Check sheet for the drawn part. Datum: minimum x, y, z corner. Units: mm. A direction names the side the tool comes from. Give positions to 0.01 mm unless a question says otherwise; leave off trailing zeros. Loops run counter-clockwise (first coordinate to the right, second up) from the corner with the lowest first, then second, coordinate; pieces in that order, holes last.
1. Cross-section at B-B, the plane y = 9.5. Record the cut outline in (x, z).
2. Material ranges on L1, parallel to Z at x = 21, y = 1.05; L2, parallel to X at y = 15.3, z = 13 (1 decimal); L3, parallel to Y at x = 3.5, z = 19, recorded low to high.
3. Go/stop test with flat-tipped pins: pin 1 Ø6 at (x, z) = (34.86, 13) entering from -Y; pin 2 Ø3 at (x, y) = (23.5, 7) entering from +Z; pin 3 Ø6 at (x, y) = (9.5, 7.5) entering from +Z. Record where each tip stops, or that it passes through.
4. Tool access check on the marked faces 1 and 2. Record the directions out of +Z, -Z, +X, -X, +Y, -Y that give a thin tool (end or side, any length) a straight path to the whole face; none if there is none.
5. Cross-section at A-A, the plane z = 21. Record the cut outline in (x, y).
6. Release check for a two-part mould opening along X. For the marked faces 3 and 4 record: +X half, -X half, draft (parallel to the pull), parting line (faces both ways), or undercut.
7. Cross-section at C-C, the plane z = 36. State how many separate pieces and enclosed holes the cut face has, plus the area to 3 significant figures.
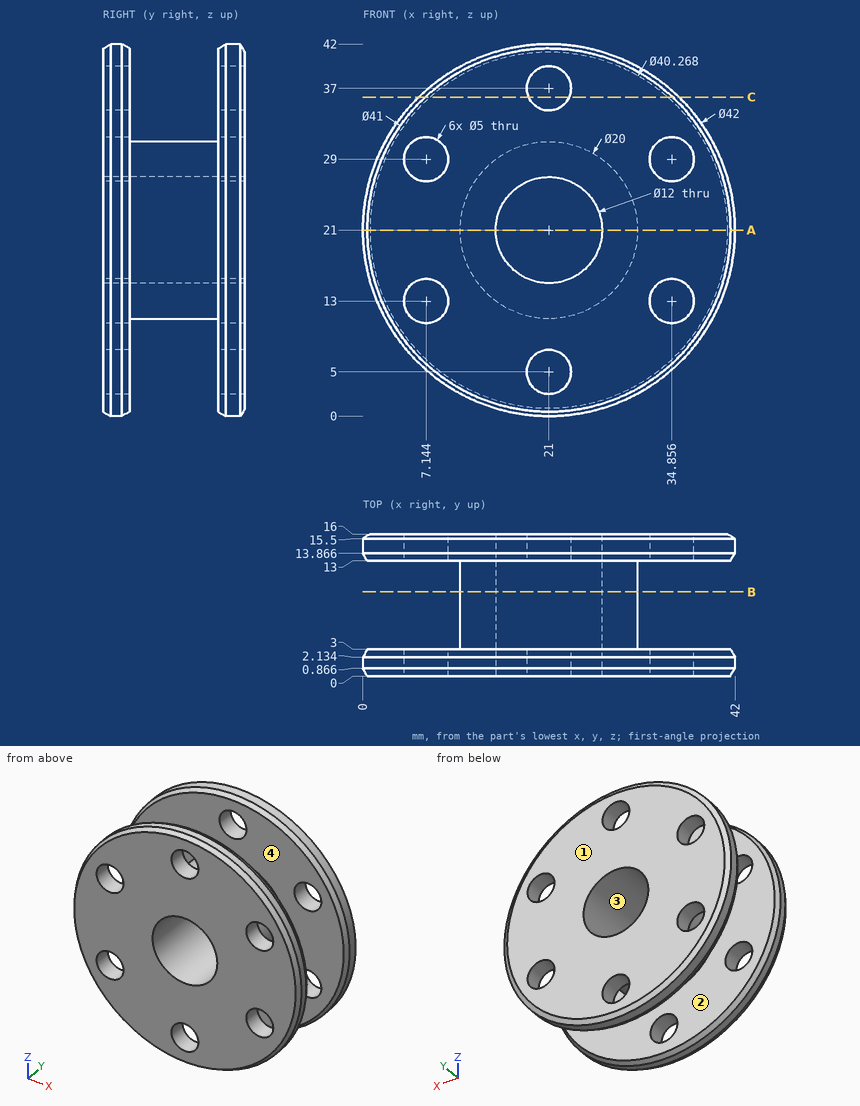
Result:
1. outline: circle Ø20 at (21, 21); hole circle Ø12 at (21, 21)
2. L1: z = 0 to 2.5, 7.5 to 15, 27 to 34.5, 39.5 to 42
2. L2: x = 1.6 to 4.6, 9.6 to 32.4, 37.4 to 40.4
2. L3: y = 0 to 3, 13 to 16
3. pin 1: stops at y = 0
3. pin 2: stops at z = 30.95
3. pin 3: stops at z = 26.27
4. face 1: +Z, -Z, +X, -X, +Y
4. face 2: none
5. outline: (0, 0.87) - (0.5, 0) - (15, 0) - (15, 16) - (0.87, 16) - (0, 15.5) - (0, 13.87) - (0.5, 13) - (11, 13) - (11, 3) - (0.5, 3) - (0, 2.13) - close; (27, 0) - (41.5, 0) - (42, 0.87) - (42, 2.13) - (41.5, 3) - (31, 3) - (31, 13) - (41.5, 13) - (42, 13.87) - (42, 15.5) - (41.13, 16) - (27, 16) - close
6. face 3: undercut
6. face 4: draft
7. separate pieces: 4
7. enclosed holes: 0
7. area: 146 mm2
